Source: three-view drawing plus pictorial views. Frame: mm from the lowest corner of the part. Round coordinates to 2 decimals unless told otherwise and drop trailing zeros. Write each loop counter-clockwise with the first axis right and the second up, starting at its lowest first coordinate (ties: lowest second). Pieces come first, ordered by that corner, then holes.
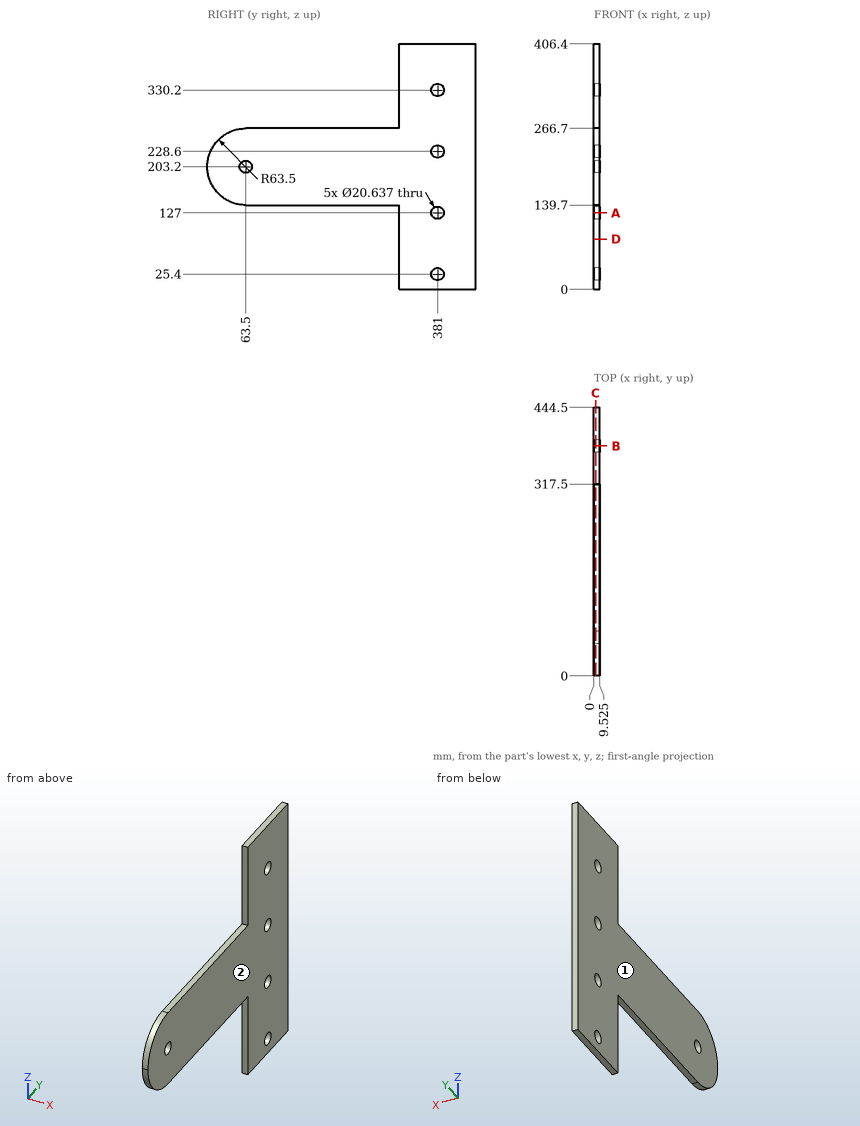
1) Section C-C on x = 3. State how many separate pieces and enclosed holes the cut face has, plus the area to 3 significant figures.
2) First-contact query: P1, Ø5, axis at x = 6, z = 353.5, coming from the -Y side. Flat tip, straight axial feed; report the tip coordinate or a pass-through.
3) Draft query along X for the marked faces 1 and 2. Return one class per face: pulls with the +X half, pulls with the -X half, needs draft (parallel to the pull), parting line crosses it, or undercut.
4) Line query: probe 1 along Z at (x, y) = (7.25, 381); probe 2 along Z at (x, y) = (0.5, 287); probe 3 along Y at (x, z) = (4.5, 328). Output: solid intervals per line, ascending.
5) Section A-A on z = 127. Output: boundary loops of the cut face in (x, y) (1 decimal).
6) Section B-B on y = 381. Output: boundary loops of the cut face in (x, z) (1 decimal).
7) Section D-D on z = 83.5. Output: boundary loops of the cut face in (x, y) (1 decimal).
Filled in:
1. separate pieces: 1
1. enclosed holes: 5
1. area: 88,500 mm2
2. P1: stops at y = 317.5
3. face 1: pulls with the -X half
3. face 2: pulls with the +X half
4. probe 1: z = 0 to 15.08, 35.72 to 116.68, 137.32 to 218.28, 238.92 to 319.88, 340.52 to 406.4
4. probe 2: z = 139.7 to 266.7
4. probe 3: y = 317.5 to 370.92, 391.08 to 444.5
5. outline: (0, 317.5) - (9.5, 317.5) - (9.5, 370.7) - (0, 370.7) - close; (0, 391.3) - (9.5, 391.3) - (9.5, 444.5) - (0, 444.5) - close
6. outline: (0, 0) - (9.5, 0) - (9.5, 15.1) - (0, 15.1) - close; (0, 35.7) - (9.5, 35.7) - (9.5, 116.7) - (0, 116.7) - close; (0, 137.3) - (9.5, 137.3) - (9.5, 218.3) - (0, 218.3) - close; (0, 238.9) - (9.5, 238.9) - (9.5, 319.9) - (0, 319.9) - close; (0, 340.5) - (9.5, 340.5) - (9.5, 406.4) - (0, 406.4) - close
7. outline: (0, 317.5) - (9.5, 317.5) - (9.5, 444.5) - (0, 444.5) - close
